from build123d import *

# Parameters (mm, degrees)
F0_W     = 50.8
F0_H     = 50.8
F1_DEPTH = 50.8
F3_DEPTH = 25.4
F5_DEPTH = 25.4


with BuildPart() as f1:
    # F0 (on Front) → F1 (new body)
    with BuildSketch(Plane.XZ):
        with Locations((-30.37813, -8.567312)):
            Rectangle(F0_W, F0_H)
    extrude(amount=-F1_DEPTH)

    # F2 (on Front) → F3 (cut)
    with BuildSketch(Plane.XZ):
        Polygon((-43.071337, -13.54893), (-4.849092, -13.54893), (-5.134332, 16.686577), (-43.071337, 16.686577), align=None)
    extrude(amount=-F3_DEPTH, mode=Mode.SUBTRACT)

    # F4 (on Front) → F5 (cut)
    with BuildSketch(Plane.XZ):
        Polygon((-4.563851, 16.971819), (-42.786095, 16.971819), (-41.930374, -12.122728), (-4.563851, -12.122728), align=None)
    extrude(amount=-F5_DEPTH, mode=Mode.SUBTRACT)


solid = f1.part
Input: part model. Units: mm. Frame: model coordinates. Give positions to 0.01 mm unless a question says otherwise; leave off trailing zeros. Loops run counter-clockwise (first coordinate to the right, second up) from the corner with the lowest first, then second, coordinate; pieces in that order, holes last. Notation, with made-up numbers: (-13, 56.25) -> (22, 56.25) arc R29 cw to (22, 80.25) -> close; hole circle Ø3 at (44, 47.25). An arc over 180 degrees is marked (long way). Answer as a JSON object with one key per item and string values. Group by question number.
Item 1: Pull-direction query (Z, two-part tool) for faces 1 (the flat face through (-43.071, 13, 2)), 2 (the flat face through (-31, 25, -33.967)), 3 (the flat face through (-55.778, 25, -9)); classes: released by +Z, released by -Z, zero draft, split by the parting line, or undercut.
Item 2: Cut plane B-B, the plane y = 6. Return the cut outline in (x, z), and give its area (3 significant figures).
Item 3: Pin query (flat end, axial travel): P1, Ø7.5, axis at y = 16, z = 3, coming from the +X side; P2, Ø24.5, axis at x = -17.5, z = 3, coming from the -Y side; P3, Ø12, axis at x = -13.5, y = 17, coming from the +Z side. Return the tip coordinate at first contact, or that it passes through.
Item 4: Cut plane C-C, the plane z = -7. Return the cut outline in (x, y), and give its area (3 significant figures).
Item 5: Cut plane A-A, the plane x = -13. Return the cut outline in (y, z).
Item 6: Line query: probe 1 along X at (y, z) = (3.5, 0.5); probe 2 along Y at (x, z) = (-43, 14); probe 3 along Z at (x, y) = (-11.5, 12). Output: solid intervals per line, ascending.
Checks:
{
 "1": {"face 1": "undercut", "face 2": "released by -Z", "face 3": "zero draft"},
 "2": {"outline": "(-55.78, -33.97) -> (-4.98, -33.97) -> (-4.98, -13.55) -> (-43.07, -13.55) -> (-43.07, 16.69) -> (-42.78, 16.69) -> (-42.78, 16.83) -> (-55.78, 16.83) -> close", "area": "1,420 mm²"},
 "3": {"P1": "stops at x = -43.07", "P2": "stops at y = 25.4", "P3": "stops at z = -13.55"},
 "4": {"outline": "(-55.78, 0) -> (-43.07, 0) -> (-43.07, 25.4) -> (-4.98, 25.4) -> (-4.98, 50.8) -> (-55.78, 50.8) -> close", "area": "1,610 mm²"},
 "5": {"outline": "(0, -33.97) -> (50.8, -33.97) -> (50.8, 16.83) -> (25.4, 16.83) -> (25.4, -13.55) -> (0, -13.55) -> close"},
 "6": {"probe 1": "x = -55.78 to -43.07", "probe 2": "y = 25.4 to 50.8", "probe 3": "z = -33.97 to -13.55"}
}
